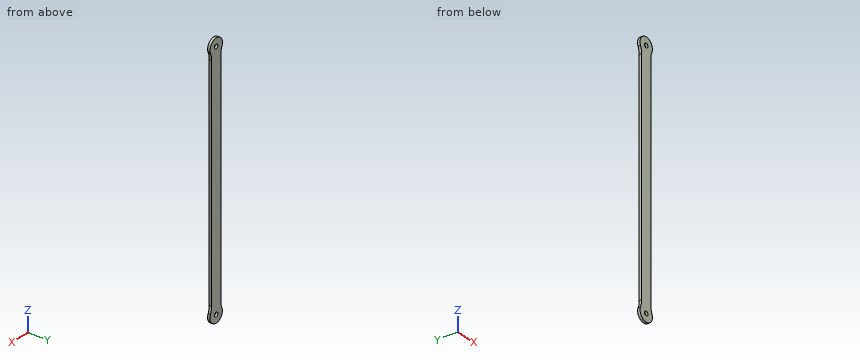
Autodesk Inventor part; units mm, degrees
ref_plane "YZ Plane" through (0, 0, 0) normal (1, 0, 0) x (0, 1, 0)
ref_plane "XZ Plane" through (0, 0, 0) normal (0, 1, 0) x (-1, 0, 0)
ref_plane "XY Plane" through (0, 0, 0) normal (0, 0, 1) x (1, 0, 0)
sketch "Sketch1" plane through (0, 0, 0) normal (0, 1, 0) x (-1, 0, 0)
  arc A0 (5.0015, -2.165) -> (-5.0015, -2.165) centre (0, 0) ccw
  line L0 (4, -7) -> (4, -163)
  line L1 (-4, -7) -> (-4, -163)
  arc A1 (5.0015, -2.165) -> (4, -7) centre (16.1716, -7) ccw
  arc A2 (-4, -7) -> (-5.0015, -2.165) centre (-16.1716, -7) ccw
  arc A3 (-5.0015, -167.835) -> (5.0015, -167.835) centre (0, -170) ccw
  arc A4 (4, -163) -> (5.0015, -167.835) centre (16.1716, -163) ccw
  arc A5 (-5.0015, -167.835) -> (-4, -163) centre (-16.1716, -163) ccw
  dimension "d0" = 10.9
  dimension "d4" = 4
  dimension "d5" = 4
  dimension "d6" = 0
  dimension "d7" = 10.9
  dimension "d8" = 170
  dimension "d9" = 0
  dimension "d10" = 7
  dimension "d12" = 4
  dimension "d13" = 7
extrude "Extrusion1" add sketch "Sketch1" along normal blind 1.7
sketch "Sketch2" plane through (0, 1.7, 0) normal (0, 1, 0) x (1, 0, 0)
  arc A0 (5.0015, 167.835) -> (-5.0015, 167.835) centre (0, 170) ccw
  arc A1 (-5.0015, 2.165) -> (5.0015, 2.165) centre (0, 0) ccw
  circle A2 centre (0, 0) radius 1.5
  circle A3 centre (0, 170) radius 1.5
  dimension "d16" = 3
  dimension "d17" = 3
extrude "Extrusion2" cut sketch "Sketch2" against normal blind 1.7
equation "\"BendRadius\" = Thickness"
equation "\"BendReliefWidth\" = Thickness"
equation "\"BendReliefDepth\" = 0.5 * Thickness"
equation "\"CornerReliefSize\" = 4 * Thickness"
equation "\"MinimumRemnant\" = 2 * Thickness"
equation "\"TransitionRadius\" = BendRadius"
equation "\"JacobiRadiusSize\" = BendRadius"
equation "\"GapSize\" = Thickness"
properties part number "A2P1"
Verification items for the finished model (mm, model axes). Round coordinates to 2 decimals unless told otherwise and drop trailing zeros. Loops run counter-clockwise (first coordinate to the right, second up) from the corner with the lowest first, then second, coordinate; pieces in that order, holes last. Notation, with made-up numbers: (1.5, 5) -> (49.5, 5) arc R14 cw to (49.5, 18) -> close; hole circle Ø5 at (-10.75, -29). An arc over 180 degrees is marked (long way). Answer as a JSON object with one key per item and string values.
Q1. Scan lines: line 1 (X direction, y = 1.3, z = 0); line 2 (Z direction, x = -1.25, y = 0.9); line 3 (X direction, y = 0.1, z = -58). Record each from-to range of solid material in increasing order. Write a range as from..to.
Data:
{"line 1": "x = -5.45..-1.5, 1.5..5.45", "line 2": "z = -175.3..-170.83, -169.17..-0.83, 0.83..5.3", "line 3": "x = -4..4"}
Q2. Section check D-D (z = -45). Record the boundary of the cut face in (x, y).
Data:
{"outline": "(-4, 0) -> (4, 0) -> (4, 1.7) -> (-4, 1.7) -> close"}
Q3. Section check A-A (z = 0). Record the boundary of the cut face in (x, y), then the cut area to 3 significant figures.
Data:
{"outline": "(-5.45, 0) -> (-1.5, 0) -> (-1.5, 1.7) -> (-5.45, 1.7) -> close; (1.5, 0) -> (5.45, 0) -> (5.45, 1.7) -> (1.5, 1.7) -> close", "area": "13.4 mm2"}
Q4. Section check B-B (x = 0). Record the boundary of the cut face in (y, z), then the cut area to 3 significant figures.
Data:
{"outline": "(0, -175.45) -> (1.7, -175.45) -> (1.7, -171.5) -> (0, -171.5) -> close; (0, -168.5) -> (1.7, -168.5) -> (1.7, -1.5) -> (0, -1.5) -> close; (0, 1.5) -> (1.7, 1.5) -> (1.7, 5.45) -> (0, 5.45) -> close", "area": "297 mm2"}
Q5. Go/stop test with a flat-tipped pin: P1, Ø0.5, axis at y = 1, z = -64.5, coming from the -X side. Record where the tip stops, or that it passes through.
Data:
{"P1": "stops at x = -4"}
Q6. Section check C-C (y = 1.05). Record the boundary of the cut face in (x, z) (1 decimal), then the cut area to 3 significant figures.
Data:
{"outline": "(-5, -167.8) arc R5.4 ccw (long way) to (5, -167.8) arc R12.2 cw to (4, -163) -> (4, -7) arc R12.2 cw to (5, -2.2) arc R5.4 ccw (long way) to (-5, -2.2) arc R12.2 cw to (-4, -7) -> (-4, -163) arc R12.2 cw to start; hole circle Ø3 at (0, -170); hole circle Ø3 at (0, 0)", "area": "1,460 mm2"}
